The listing builds one solid part. Answer for the finished solid, in the listing's coordinates (mm). A direction names the side the tool comes from. Give positions to 0.01 mm unless a question says otherwise; leave off trailing zeros. Loops run counter-clockwise (first coordinate to the right, second up) from the corner with the lowest first, then second, coordinate; pieces in that order, holes last. Notation, with made-up numbers: (84, 27.5) - (122, 27.5) arc R8 cw to (122, 38.5) - close; hole circle Ø3 at (12.5, -32). An arc over 180 degrees is marked (long way). Write item = value, one per line. Start each with the question number.
1) The part is cut by section C-C on x = 51. Write down the section's boundary in (y, z), plus the area to 3 significant figures.
2) Flat-ended cylindrical pins translate along their axes: P1, Ø1.5, axis at x = 48.5, y = 4, coming from the -Z side; P2, Ø2, axis at x = 82, y = 3.5, coming from the -Z side; P3, Ø2, axis at y = 2, z = -14, coming from the -X side. Find the tip coordinate at first contact, or state that the pin passes through.
3) Which of the six approach directions +Z, -Z, +X, -X, +Y, -Y give full straight-line access (tool end or side, diameter ignored) to faces 4 (the flat face through (110, 3, 28)), 5 (the flat face through (-70, 3, 34.9))?
4) The part is cut by section A-A on x = 25. Write down the section's boundary in (y, z), plus the area to 3 significant figures.
5) The part is cut by section B-B on z = 12.5. Write down the section's boundary in (x, y).
6) The mould has two halves that part along Z. Classify faces 1 (the flat face through (70, 3, 9.9)), 2 (the flat face through (14, 3, 9.5)), 3 (the flat face through (2, 6, 15)): +Z half, -Z half, draft (parallel to the pull), parting line (faces both ways), or undercut.
7) Consider probe 1 along X at (y, z) = (2.45, -4); probe 2 along Z at (x, y) = (14.5, 3.35); probe 3 along Z at (x, y) = (80, 1.35). Determine where each line is inside the solid, lowest interval first.
8) The part is cut by section D-D on z = -43. Write down the section's boundary in (x, y), plus the area to 3 significant figures.
Autodesk Inventor part; units mm, degrees
ref_plane "YZ Plane" through (0, 0, 0) normal (1, 0, 0) x (0, 1, 0)
ref_plane "XZ Plane" through (0, 0, 0) normal (0, 1, 0) x (-1, 0, 0)
ref_plane "XY Plane" through (0, 0, 0) normal (0, 0, 1) x (1, 0, 0)
sketch "Sketch2" plane through (0, 0, 0) normal (0, 1, 0) x (-1, 0, 0)
  line L0 (110, 62.5) -> (-110, 62.5)
  line L1 (-110, 62.5) -> (-110, -62.5)
  line L2 (-110, -62.5) -> (110, -62.5)
  line L3 (110, -62.5) -> (110, 62.5)
  line L4 (110, 62.5) -> (-110, -62.5) construction
  line L5 (-110, 62.5) -> (110, -62.5) construction
  line L6 (11.5, -50.5) -> (17.5, -50.5)
  line L7 (17.5, -50.5) -> (17.5, -38.5)
  line L8 (17.5, -38.5) -> (11.5, -38.5)
  line L9 (11.5, -38.5) -> (11.5, -50.5)
  line L10 (11.5, -26.5) -> (17.5, -26.5)
  line L11 (17.5, -26.5) -> (17.5, -14.5)
  line L12 (17.5, -14.5) -> (11.5, -14.5)
  line L13 (11.5, -14.5) -> (11.5, -26.5)
  line L14 (11.5, -2.5) -> (17.5, -2.5)
  line L15 (17.5, -2.5) -> (17.5, 9.5)
  line L16 (17.5, 9.5) -> (11.5, 9.5)
  line L17 (11.5, 9.5) -> (11.5, -2.5)
  line L18 (-17.5, -50.5) -> (-11.5, -50.5)
  line L19 (-11.5, -50.5) -> (-11.5, -38.5)
  line L20 (-11.5, -38.5) -> (-17.5, -38.5)
  line L21 (-17.5, -38.5) -> (-17.5, -50.5)
  line L22 (-17.5, -26.5) -> (-11.5, -26.5)
  line L23 (-11.5, -26.5) -> (-11.5, -14.5)
  line L24 (-11.5, -14.5) -> (-17.5, -14.5)
  line L25 (-17.5, -14.5) -> (-17.5, -26.5)
  line L26 (-17.5, -2.5) -> (-11.5, -2.5)
  line L27 (-11.5, -2.5) -> (-11.5, 9.5)
  line L28 (-11.5, 9.5) -> (-17.5, 9.5)
  line L29 (-17.5, 9.5) -> (-17.5, -2.5)
  line L30 (0, 0) -> (0, -18.9718)
  line L31 (25, -2.5) -> (25, -52.5) construction
  line L32 (22.4, -2.5) -> (22.4, -52.5)
  line L33 (27.6, -52.5) -> (27.6, -2.5)
  arc A0 (27.6, -2.5) -> (22.4, -2.5) centre (25, -2.5) ccw
  arc A1 (22.4, -52.5) -> (27.6, -52.5) centre (25, -52.5) ccw
  line L34 (100, 12.5) -> (40, 12.5) construction
  line L35 (100, 15.1) -> (40, 15.1)
  line L36 (40, 9.9) -> (100, 9.9)
  arc A2 (100, 9.9) -> (100, 15.1) centre (100, 12.5) ccw
  arc A3 (40, 15.1) -> (40, 9.9) centre (40, 12.5) ccw
  line L37 (100, 37.5) -> (40, 37.5) construction
  line L38 (100, 40.1) -> (40, 40.1)
  line L39 (40, 34.9) -> (100, 34.9)
  arc A4 (100, 34.9) -> (100, 40.1) centre (100, 37.5) ccw
  arc A5 (40, 40.1) -> (40, 34.9) centre (40, 37.5) ccw
  line L40 (-25, -2.5) -> (-25, -52.5) construction
  line L41 (-22.4, -2.5) -> (-22.4, -52.5)
  line L42 (-27.6, -52.5) -> (-27.6, -2.5)
  arc A6 (-22.4, -2.5) -> (-27.6, -2.5) centre (-25, -2.5) ccw
  arc A7 (-27.6, -52.5) -> (-22.4, -52.5) centre (-25, -52.5) ccw
  line L43 (-100, 12.5) -> (-40, 12.5) construction
  line L44 (-100, 15.1) -> (-40, 15.1)
  line L45 (-40, 9.9) -> (-100, 9.9)
  arc A8 (-100, 15.1) -> (-100, 9.9) centre (-100, 12.5) ccw
  arc A9 (-40, 9.9) -> (-40, 15.1) centre (-40, 12.5) ccw
  line L46 (-100, 37.5) -> (-40, 37.5) construction
  line L47 (-100, 40.1) -> (-40, 40.1)
  line L48 (-40, 34.9) -> (-100, 34.9)
  arc A10 (-100, 40.1) -> (-100, 34.9) centre (-100, 37.5) ccw
  arc A11 (-40, 34.9) -> (-40, 40.1) centre (-40, 37.5) ccw
  circle A12 centre (80, 52.5) radius 2.6
  circle A13 centre (-80, 52.5) radius 2.6
  line L49 (110, -7.5) -> (45, -62.5)
  line L50 (-45, -62.5) -> (-110, -7.5)
  point P0 (25, -27.5)
  point P1 (70, 12.5)
  point P2 (70, 37.5)
  point P3 (-25, -27.5)
  point P4 (-70, 12.5)
  point P5 (-70, 37.5)
  dimension "d52" = 220
  dimension "d53" = 125
  dimension "d54" = 12
  dimension "d55" = 6
  dimension "d58" = 24
  dimension "d61" = 29
  dimension "d65" = 12
  dimension "d66" = 5.2
  dimension "d68" = 100
  dimension "d69" = 115
  dimension "d70" = 40
  dimension "d71" = 65
  dimension "d72" = 15
  dimension "d73" = 25
  dimension "d75" = 15
  dimension "d76" = 5.2
  dimension "d79" = 30
  dimension "d80" = 10
  dimension "d81" = 20
  dimension "d82" = 20
extrude "Extrusion2" add sketch "Sketch2" along normal blind 6 contours L3 L49 L2 L50 L1 L0
properties part number "phone_holder_back" material "Acrylic, Clear"
Answer below:
q1.outline = (0, -57.42) - (6, -57.42) - (6, 9.9) - (0, 9.9) - close; (0, 15.1) - (6, 15.1) - (6, 34.9) - (0, 34.9) - close; (0, 40.1) - (6, 40.1) - (6, 62.5) - (0, 62.5) - close
q1.area = 657 mm2
q2.P1 = -60.17
q2.P2 = -32.04
q2.P3 = -103.5
q3.face_4 = +Z, -Z, +X, +Y, -Y
q3.face_5 = +Y, -Y
q4.outline = (0, -62.5) - (6, -62.5) - (6, -55.1) - (0, -55.1) - close; (0, 0.1) - (6, 0.1) - (6, 62.5) - (0, 62.5) - close
q4.area = 419 mm2
q5.outline = (-110, 0) - (-102.6, 0) - (-102.6, 6) - (-110, 6) - close; (-37.4, 0) - (37.4, 0) - (37.4, 6) - (-37.4, 6) - close; (102.6, 0) - (110, 0) - (110, 6) - (102.6, 6) - close
q6.face_1 = undercut
q6.face_2 = undercut
q6.face_3 = draft
q7.probe_1 = -110 to -27.6, -22.4 to 22.4, 27.6 to 110
q7.probe_2 = -62.5 to -50.5, -38.5 to -26.5, -14.5 to -2.5, 9.5 to 62.5
q7.probe_3 = -32.88 to 9.9, 15.1 to 34.9, 40.1 to 49.9, 55.1 to 62.5
q8.outline = (-68.05, 0) - (-27.6, 0) - (-27.6, 6) - (-68.05, 6) - close; (-22.4, 0) - (-17.5, 0) - (-17.5, 6) - (-22.4, 6) - close; (-11.5, 0) - (11.5, 0) - (11.5, 6) - (-11.5, 6) - close; (17.5, 0) - (22.4, 0) - (22.4, 6) - (17.5, 6) - close; (27.6, 0) - (68.05, 0) - (68.05, 6) - (27.6, 6) - close
q8.area = 682 mm2
